```python
from build123d import *

# Parameters (mm, degrees)
BOSS_EXTRUDE1_DEPTH = 1
SKETCH2_R           = 1.2
SKETCH2_W           = 4.2
SKETCH2_H           = 6.5
CUT_EXTRUDE1_DEPTH  = 11
SKETCH3_W           = 37
SKETCH3_H           = 1
BOSS_EXTRUDE2_DEPTH = 11.45


with BuildPart() as part:
    # Sketch1 → Boss-Extrude1 (new body)
    with BuildSketch(Plane.XY):
        Polygon((18.5, 23.5), (18.5, 30.5), (-18.5, 30.5), (-26.5, 30.5), (-26.5, 8.5), (-18.5, 8.5), (-18.5, -23.5), (18.5, -23.5), align=None)
    extrude(amount=BOSS_EXTRUDE1_DEPTH)

    # Sketch2 → Cut-Extrude1 (cut)
    with BuildSketch(Plane.XY.offset(1)):
        with Locations((-22.5, 10.735)):
            Circle(SKETCH2_R)
        with Locations((-22.5, 28.265)):
            Circle(SKETCH2_R)
        with Locations((-22.5, 19.5)):
            Rectangle(SKETCH2_W, SKETCH2_H)
    extrude(amount=-CUT_EXTRUDE1_DEPTH, mode=Mode.SUBTRACT)

    # Sketch3 → Boss-Extrude2 (add)
    with BuildSketch(Plane(origin=(0, 0, 0), x_dir=(-1, 0, 0), z_dir=(0, 0, -1))):
        with Locations((0, -23)):
            Rectangle(SKETCH3_W, SKETCH3_H)
    extrude(amount=BOSS_EXTRUDE2_DEPTH)


solid = part.part
```
CAD build for the part. Positions are in the model's coordinates, mm. A direction names the side the tool comes from. Round coordinates to 2 decimals unless told otherwise and drop trailing zeros. Order: outer loops, then holes, each group sorted by start corner. A loop starts at its lowest first (then second) coordinate and runs counter-clockwise, first axis right, second up. Notation, with made-up numbers: (-14, 88.25) -> (36, 88.25) arc R16 ccw to (36, 103.25) -> close; hole circle Ø7 at (26, 37). An arc over 180 degrees is marked (long way). One line per question, with ' | ' between items.
Q1. Which spindle directions (+Z, -Z, +X, -X, +Y, -Y) get a long thin tool onto all of the face, cutting with end or side? Do faces 4 (the flat face through (1, 4, 0)), 5 (the flat face through (-18.5, -12.3, 0.3)), 6 (the cylindrical face through (-23.7, 10.8, 0.5)). Say none if no direction does.
Completed:
face 4: -Z, +X, -X, +Y | face 5: +Z, -Z, -X, -Y | face 6: +Z, -Z
Q2. Drop flat-ended pins along their axis: pin 1 (0.8 mm diameter, centred on x = -23, z = 0.5, fed in from -Y); pin 2 (4 mm diameter, centred on x = 9, y = -4, fed in from -Z); pin 3 (6 mm diameter, centred on y = -13.5, z = -2.5, fed in from -X); pin 4 (1.4 mm diameter, centred on x = -22.5, y = 10.735, fed in from -Z). Give the stop position or say it passes through.
Completed:
pin 1: stops at y = 8.5 | pin 2: stops at z = 0 | pin 3: stops at x = -18.5 | pin 4: passes through
Q3. Slice it at B-B (x = -22.5). Write the cut outline in (y, z) (3 decimals).
Completed:
outline: (8.5, 0) -> (9.535, 0) -> (9.535, 1) -> (8.5, 1) -> close; (11.935, 0) -> (16.25, 0) -> (16.25, 1) -> (11.935, 1) -> close; (22.75, 0) -> (27.065, 0) -> (27.065, 1) -> (22.75, 1) -> close; (29.465, 0) -> (30.5, 0) -> (30.5, 1) -> (29.465, 1) -> close
Q4. Two-plate mould, pull along Y, no slides. Class faces 1 (the flat face through (1, 4, 1)), 2 (the cylindrical face through (-23.38, 29.08, 0.51)), 3 (the flat face through (0, -22.5, -6)): released by +Y, released by -Y, zero draft, split by the parting line, or undercut.
Completed:
face 1: zero draft | face 2: undercut | face 3: released by +Y
Q5. Slice it at A-A (y = 17.5). Write the cut outline in (x, z).
Completed:
outline: (-26.5, 0) -> (-24.6, 0) -> (-24.6, 1) -> (-26.5, 1) -> close; (-20.4, 0) -> (18.5, 0) -> (18.5, 1) -> (-20.4, 1) -> close
Q6. Slice it at C-C (x = -10). Write the cut outline in (y, z).
Completed:
outline: (-23.5, -11.45) -> (-22.5, -11.45) -> (-22.5, 0) -> (30.5, 0) -> (30.5, 1) -> (-23.5, 1) -> close
Q7. Slice it at D-D (z = -2). Write the cut outline in (x, y).
Completed:
outline: (-18.5, -23.5) -> (18.5, -23.5) -> (18.5, -22.5) -> (-18.5, -22.5) -> close
Q8. Probe probe 1 along Y at (x, z) = (-22.5, 0.85) (3 decimals); probe 2 along Y at (x, z) = (-16.5, -8); probe 3 along Z at (x, y) = (-2, 16.5). List the from-to ranges inside material, lowest first.
Completed:
probe 1: y = 8.5 to 9.535, 11.935 to 16.25, 22.75 to 27.065, 29.465 to 30.5 | probe 2: y = -23.5 to -22.5 | probe 3: z = 0 to 1
